```python
from build123d import *

# Parameters (mm, degrees)
F0_R     = 2.54
F0_R_2   = 3.5687
F0_R_3   = 8.001
F1_DEPTH = 6.35
F3_R     = 3.5687
F4_DEPTH = 4.953
F4_TAPER = -45
F5_R     = 8.5217
F5_R_2   = 6.35
F6_DEPTH = 4.953


with BuildPart() as f1:
    # F0 (on Top) → F1 (new body)
    with BuildSketch(Plane.XY):
        with BuildLine():
            Line((90.7821191281, 46.4983058831), (25.955052352, 46.4983058831))
            Line((25.955052352, 46.4983058831), (-38.227, 28.1307150105))
            ThreePointArc((-38.227, 28.1307150105), (-58.928, 0), (-38.227, -28.1307150105))
            Line((-38.227, -28.1307150105), (25.955052352, -46.4983058831))
            Line((25.955052352, -46.4983058831), (90.7821191281, -46.4983058831))
            ThreePointArc((90.7821191281, -46.4983058831), (118.2538107645, 0), (90.7821191281, 46.4983058831))
        make_face()
        with Locations((25.955052352, -33.226947648)):
            Circle(F0_R, mode=Mode.SUBTRACT)
        with Locations((-38.227, -15.1779612267)):
            Circle(F0_R_2, mode=Mode.SUBTRACT)
        with Locations((92.408947648, -33.226947648)):
            Circle(F0_R, mode=Mode.SUBTRACT)
        with Locations((-38.227, 15.1779612267)):
            Circle(F0_R_2, mode=Mode.SUBTRACT)
        with Locations((-11.938, 0)):
            Circle(F0_R_2, mode=Mode.SUBTRACT)
        with BuildLine():
            ThreePointArc((22.5003193406, 3.302), (25.8023193406, 0), (22.5003193406, -3.302))
            Line((22.5003193406, -3.302), (9.7621892355, -3.302))
            ThreePointArc((9.7621892355, -3.302), (6.4601892355, 0), (9.7621892355, 3.302))
            Line((9.7621892355, 3.302), (22.5003193406, 3.302))
        make_face(mode=Mode.SUBTRACT)
        with Locations((25.955052352, 33.226947648)):
            Circle(F0_R, mode=Mode.SUBTRACT)
        with Locations((59.182, 0)):
            Circle(F0_R_3, mode=Mode.SUBTRACT)
        with BuildLine():
            ThreePointArc((95.8636806594, -3.302), (92.5616806594, 0), (95.8636806594, 3.302))
            Line((95.8636806594, 3.302), (108.6018107645, 3.302))
            ThreePointArc((108.6018107645, 3.302), (111.9038107645, 0), (108.6018107645, -3.302))
            Line((108.6018107645, -3.302), (95.8636806594, -3.302))
        make_face(mode=Mode.SUBTRACT)
        with Locations((92.408947648, 33.226947648)):
            Circle(F0_R, mode=Mode.SUBTRACT)
    extrude(amount=-F1_DEPTH)

    # F3 (on offset) → F4 (cut, through all)
    with BuildSketch(Plane(origin=(0, 0, -4.953), x_dir=(1, 0, 0), z_dir=(0, 0, -1))):
        with Locations((-38.227, 15.1779612267)):
            Circle(F3_R)
        with Locations((-38.227, -15.1779612267)):
            Circle(F3_R)
        with Locations((-11.938, 0)):
            Circle(F3_R)
    extrude(amount=-F4_DEPTH, taper=F4_TAPER, mode=Mode.SUBTRACT)

    # F5 (on face) → F6 (join, through all)
    with BuildSketch(Plane.XY):
        with Locations((-11.938, 0)):
            Circle(F5_R)
        with Locations((-11.938, 0)):
            Circle(F5_R_2, mode=Mode.SUBTRACT)
        with Locations((-38.227, 15.1779612267)):
            Circle(F5_R)
        with Locations((-38.227, 15.1779612267)):
            Circle(F5_R_2, mode=Mode.SUBTRACT)
        with Locations((-38.227, -15.1779612267)):
            Circle(F5_R)
        with Locations((-38.227, -15.1779612267)):
            Circle(F5_R_2, mode=Mode.SUBTRACT)
    extrude(amount=-F6_DEPTH)


solid = f1.part
```
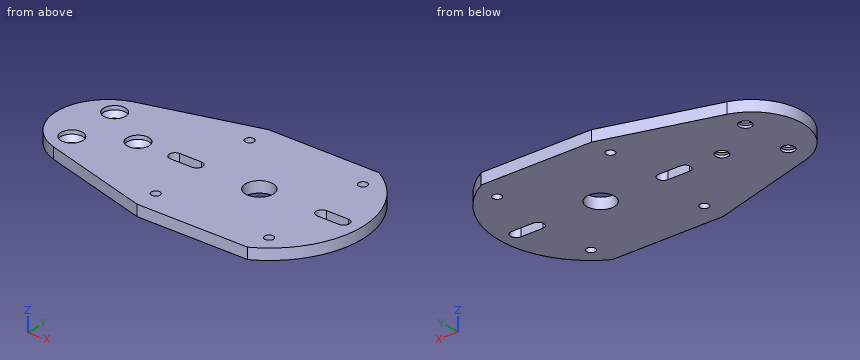
For this review, take the finished solid that the model builds, in its own axes (mm). Round coordinates to 2 decimals unless told otherwise and drop trailing zeros. Write each loop counter-clockwise with the first axis right and the second up, starting at its lowest first coordinate (ties: lowest second). Pieces come first, ordered by that corner, then holes. Notation, with made-up numbers: (-23, 44) -> (6, 44) arc R21 cw to (6, 81) -> close; hole circle Ø1 at (14, 55.5). An arc over 180 degrees is marked (long way). Use one line per item in the form item = value.
Q1. Clearance check with flat-ended pins moving along their axes: pin 1 Ø11.5 at (x, y) = (-38.23, 15.18) entering from +Z; pin 2 Ø2 at (y, z) = (-23.5, -2.5) entering from -X; pin 3 Ø7.5 at (x, y) = (-38.23, -15.18) entering from +Z; pin 4 Ø5.5 at (x, y) = (-11.938, 0) entering from +Z. State where each tip first meets the part, or that it passes through.
Resolved:
pin_1 = -2.77
pin_2 = -48.49
pin_3 = -4.77
pin_4 = through
Q2. Consider section B-B (x = 58.5). State the section outline as (y, z) points, then the cut area to 3 significant figures.
Resolved:
outline = (-46.5, -6.35) -> (-7.97, -6.35) -> (-7.97, 0) -> (-46.5, 0) -> close; (7.97, -6.35) -> (46.5, -6.35) -> (46.5, 0) -> (7.97, 0) -> close
area = 489 mm²
Q3. Consider section A-A (y = 0). State how many separate pieces and enclosed holes the cut face has, then the cut area to 3 significant figures.
Resolved:
separate_pieces = 5
enclosed_holes = 0
area = 713 mm²
Q4. To check wall thickness, follow probe 1 along Y at (x, z) = (-43, -2.5); probe 2 along X at (y, z) = (3, -3.75); probe 3 along Y at (x, z) = (-11, -1.25). State the ranges of each line that lie inside material, in increasing order. Write a range as from..to.
Resolved:
probe_1 = -26.17..-18.85, -11.51..11.51, 18.85..26.17
probe_2 = -58.77..-15.65, -8.23..8.38, 23.88..51.76, 66.6..94.48, 109.98..118.17
probe_3 = -35.92..-6.28, 6.28..35.92
Q5. Consider section D-D (x = 20). State the section outline as (y, z) points.
Resolved:
outline = (-44.79, -6.35) -> (-3.3, -6.35) -> (-3.3, 0) -> (-44.79, 0) -> close; (3.3, -6.35) -> (44.79, -6.35) -> (44.79, 0) -> (3.3, 0) -> close
